For this review, use the dimensioned drawing (mm, ordinates from the lowest corner) and the shaded views. Round coordinates to 2 decimals unless told otherwise and drop trailing zeros. Loops run counter-clockwise (first coordinate to the right, second up) from the corner with the lowest first, then second, coordinate; pieces in that order, holes last. Notation, with made-up numbers: M 0,41 L 41,41 A23 ccw 41,63 Z; hole C -27.5,23.5 d3. An arc over 180 degrees is marked long. Answer as a JSON object with one key per item and string values. Group by question number.
Item 1: To check wall thickness, follow line 1 (Z direction, x = 6.35, y = 3.25) (1 decimal); line 2 (X direction, y = 3.5, z = 89) (1 decimal); line 3 (Z direction, x = 70.5, y = 3.05) (1 decimal). State the ranges of each line that lie inside material, in increasing order.
Item 2: Consider section B-B (x = 6.35). Give the boundary of the cut face in (y, z).
Item 3: Consider section C-C (z = 6.35). Give the boundary of the cut face in (x, y).
Item 4: Consider section D-D (x = 40.5). Give the boundary of the cut face in (y, z).
Item 5: Consider section A-A (y = 1.85). State how many separate pieces and enclosed holes the cut face has, and give its area (3 significant figures).
Item 6: Insertion check: P1, Ø3, axis at x = 75, y = 3.5, coming from the -Z side; P2, Ø3, axis at y = 1, z = 59, coming from the +X side (1 decimal); P3, Ø2, axis at x = 31.5, y = 2, coming from the -Z side (1 decimal). Each pin has a flat end and moves straight along its axis. Give the tip position at first contact, or say it passes through.
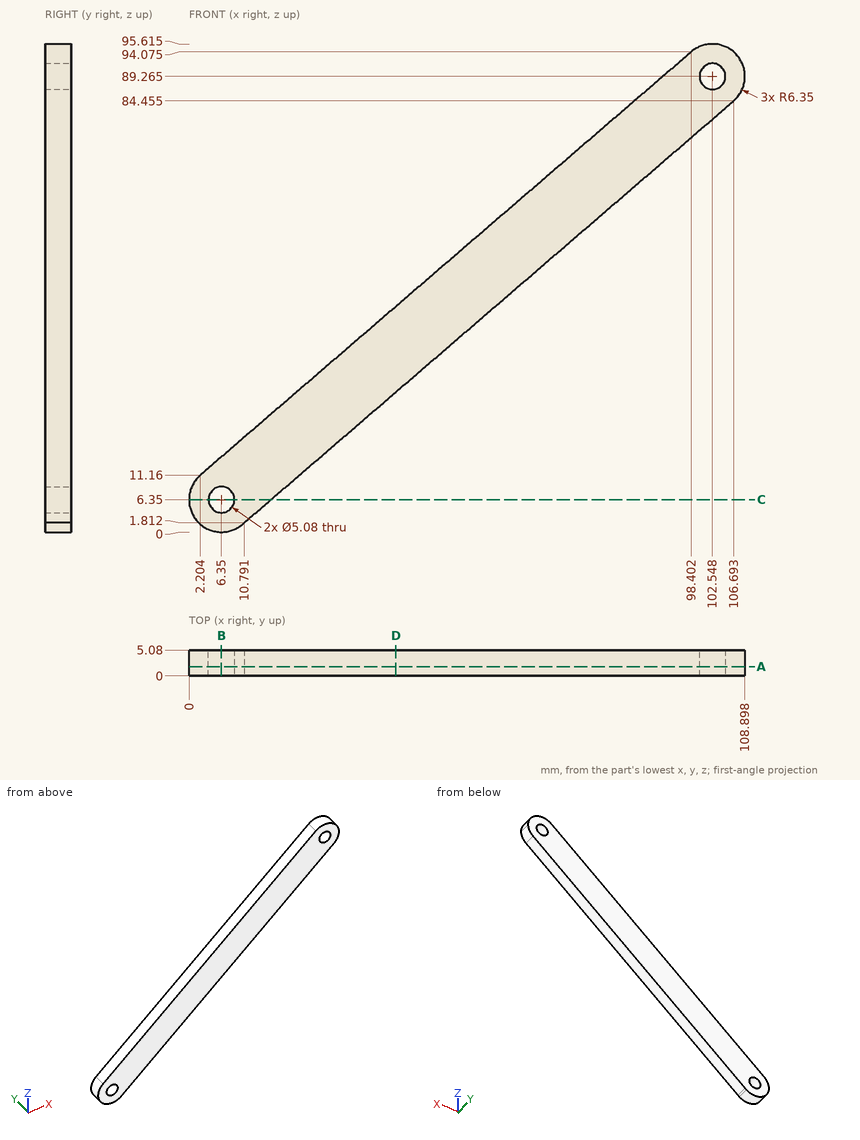
Geometry results:
{
 "1": {"line 1": "z = 0 to 3.8, 8.9 to 14.7", "line 2": "x = 92.5 to 100, 105.1 to 108.9", "line 3": "z = 53.3 to 70"},
 "2": {"outline": "M 0,0 L 5.08,0 L 5.08,3.81 L 0,3.81 Z; M 0,8.89 L 5.08,8.89 L 5.08,14.73 L 0,14.73 Z"},
 "3": {"outline": "M 0,0 L 3.81,0 L 3.81,5.08 L 0,5.08 Z; M 8.89,0 L 16.06,0 L 16.06,5.08 L 8.89,5.08 Z"},
 "4": {"outline": "M 0,27.41 L 5.08,27.41 L 5.08,44.17 L 0,44.17 Z"},
 "5": {"separate pieces": "1", "enclosed holes": "2", "area": "1,700 mm^2"},
 "6": {"P1": "stops at z = 55.85", "P2": "stops at x = 78.9", "P3": "stops at z = 18.8"}
}
